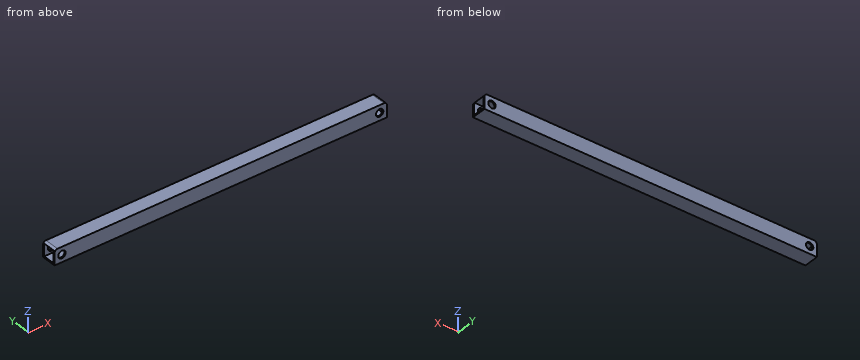
from build123d import *

# Parameters (mm, degrees)
F0_W        = 20
F0_H        = 20
F0_W_2      = 16
F0_H_2      = 16
F1_DEPTH    = 450
F2_R        = 5
F3_DEPTH    = 20.001
F4_R        = 5
F5_DEPTH    = 20.001
F6_T1_DEPTH = 40
F7_T1_DEPTH = 40


# Not quite as in the source:
# - a fillet or chamfer that OpenCascade refuses, or shapes differently, is made with other operations: its cross-section is extruded or revolved along the edge and cut away or added


with BuildPart() as f1:
    # F0 (on Right) → F1 (new body)
    with BuildSketch(Plane.YZ):
        with Locations((10, 10)):
            Rectangle(F0_W, F0_H)
        with Locations((10, 10)):
            Rectangle(F0_W_2, F0_H_2, mode=Mode.SUBTRACT)
    extrude(amount=F1_DEPTH)

    # F2 (on face) → F3 (cut, through all)
    with BuildSketch(Plane.XZ):
        with Locations((440, 10)):
            Circle(F2_R)
    extrude(amount=-F3_DEPTH, mode=Mode.SUBTRACT)

    # F4 (on face) → F5 (cut, through all)
    with BuildSketch(Plane.XZ):
        with Locations((10, 10)):
            Circle(F4_R)
    extrude(amount=-F5_DEPTH, mode=Mode.SUBTRACT)

    # F6: fillet of radius 4 on 1 edges, made by hand

    # F6_s2 → F6_t1 (cut)
    with BuildSketch(Plane.XZ.offset(-30)):
        with BuildLine():
            ThreePointArc((446, 20), (448.8284271247, 18.8284271247), (450, 16))
            Line((450, 16), (450, 20))
            Line((450, 20), (446, 20))
        make_face()
    extrude(amount=F6_T1_DEPTH, mode=Mode.SUBTRACT)

    # F7: fillet of radius 4 on 1 edges, made by hand

    # F7_s2 → F7_t1 (cut)
    with BuildSketch(Plane.XZ.offset(-30)):
        with BuildLine():
            ThreePointArc((0, 16), (1.1715728753, 18.8284271247), (4, 20))
            Line((4, 20), (0, 20))
            Line((0, 20), (0, 16))
        make_face()
    extrude(amount=F7_T1_DEPTH, mode=Mode.SUBTRACT)


solid = f1.part
Work out the finished part from the listing and answer in its coordinate system (mm). Give positions to 0.01 mm unless a question says otherwise; leave off trailing zeros. Order: outer loops, then holes, each group sorted by start corner. A loop starts at its lowest first (then second) coordinate and runs counter-clockwise, first axis right, second up. Notation, with made-up numbers: (-32.75, 11) -> (-20.75, 11) arc R15 ccw to (-20.75, 38) -> close; hole circle Ø7 at (78, -13). An arc over 180 degrees is marked (long way). One line per item, written item: value.
Item 1: Straight lines are drawn through the part: probe 1 along Z at (x, y) = (269, 10.5); probe 2 along Z at (x, y) = (440, 0.55). For each, find the intervals that lie inside material, in ascending order.
Answer sheet:
probe 1: 0 to 2, 18 to 20
probe 2: 0 to 5, 15 to 20
Item 2: Find section D-D, the plane y = 6.5. Give the vertices of the cut face in (x, z).
Answer sheet:
outline: (0, 0) -> (450, 0) -> (450, 2) -> (0, 2) -> close; (0.54, 18) -> (449.46, 18) arc R4 ccw to (446, 20) -> (4, 20) arc R4 ccw to start
Item 3: Find section C-C, the plane x = 178. Give the vertices of the cut face in (y, z), plus the area to 3 significant figures.
Answer sheet:
outline: (0, 0) -> (20, 0) -> (20, 20) -> (0, 20) -> close; hole (2, 2) -> (18, 2) -> (18, 18) -> (2, 18) -> close
area: 144 mm²
Item 4: Find section B-B, the plane x = 440. Give the vertices of the cut face in (y, z).
Answer sheet:
outline: (0, 0) -> (20, 0) -> (20, 5) -> (18, 5) -> (18, 2) -> (2, 2) -> (2, 5) -> (0, 5) -> close; (0, 15) -> (2, 15) -> (2, 18) -> (18, 18) -> (18, 15) -> (20, 15) -> (20, 20) -> (0, 20) -> close
Item 5: Find section A-A, the plane z = 10. Give the vertices of the cut face in (x, y).
Answer sheet:
outline: (0, 0) -> (5, 0) -> (5, 2) -> (0, 2) -> close; (0, 18) -> (5, 18) -> (5, 20) -> (0, 20) -> close; (15, 0) -> (435, 0) -> (435, 2) -> (15, 2) -> close; (15, 18) -> (435, 18) -> (435, 20) -> (15, 20) -> close; (445, 0) -> (450, 0) -> (450, 2) -> (445, 2) -> close; (445, 18) -> (450, 18) -> (450, 20) -> (445, 20) -> close
